Geometry check sheet. Reference: drawing and pictorial views, mm from the part's lowest x, y, z. A direction names the side the tool comes from. Give positions to 0.01 mm unless a question says otherwise; leave off trailing zeros. Order: outer loops, then holes, each group sorted by start corner. A loop starts at its lowest first (then second) coordinate and runs counter-clockwise, first axis right, second up.
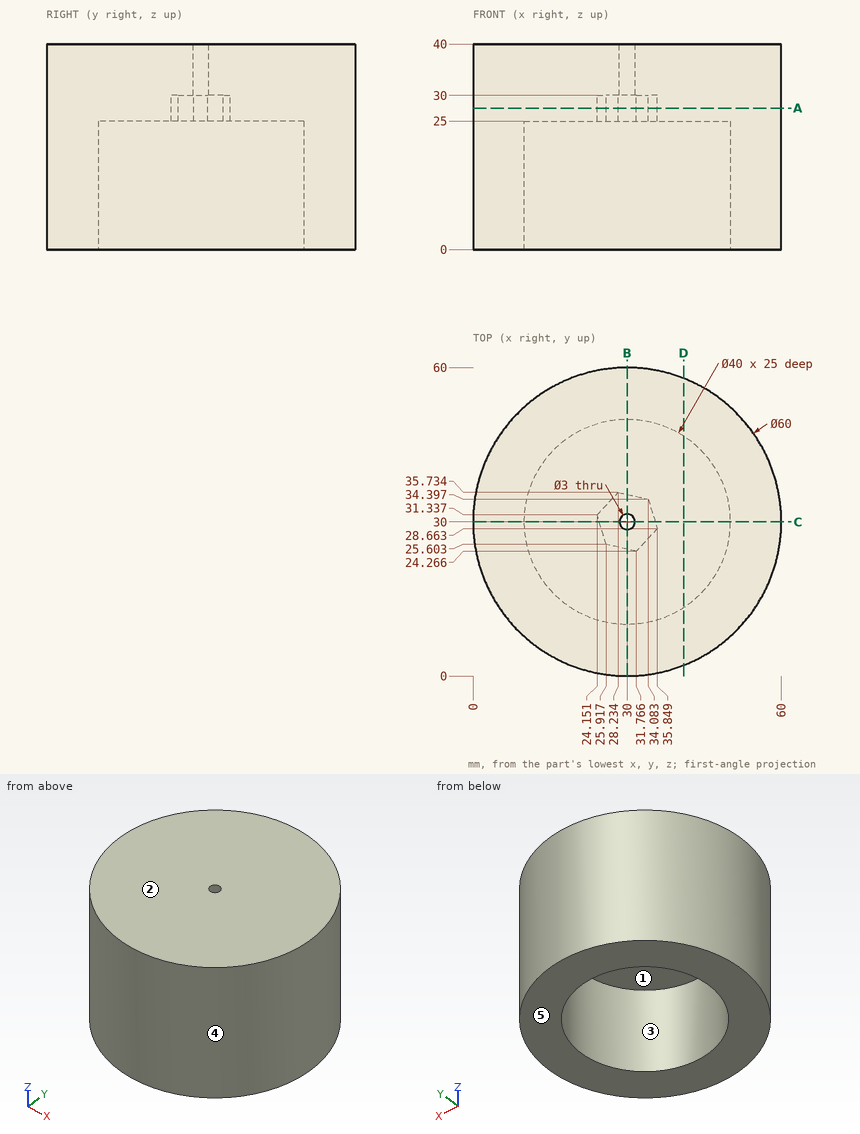
(1) Sectioned sample at B-B (x = 30). Enter the section's corners in (y, z).
(2) Sectioned sample at C-C (y = 30). Enter the section's corners in (x, z), plus the area to 3 significant figures.
(3) Thickness scan on L1, parallel to Y at x = 30, z = 8; L2, parallel to Z at x = 20.5, y = 32; L3, parallel to X at y = 21, z = 6.5. Record the ranges inside material, lowest first.
(4) Go/stop test with flat-tipped pins: P1, Ø5.5, axis at x = 29.5, y = 28.5, coming from the -Z side; P2, Ø5, axis at x = 31.5, z = 33.5, coming from the +Y side; P3, Ø6, axis at x = 21.5, z = 11, coming from the +Y side; P4, Ø2.5, axis at x = 30, y = 30, coming from the +Z side. Record where each tip stops, or that it passes through.
(5) Tool access check on the marked faces 1 and 2. Record the directions out of +Z, -Z, +X, -X, +Y, -Y that give a thin tool (end or side, any length) a straight path to the whole face; none if there is none.
(6) Sectioned sample at A-A (z = 27.5). Enter the section's corners in (x, y) (1 decimal), plus the area to 3 significant figures.
(7) Sectioned sample at D-D (x = 41). Enter the section's corners in (y, z).
(8) Release check for a two-part mould opening along Y. For the marked faces 3, 4 and 5 record: released by +Y, released by -Y, zero draft, split by the parting line, or undercut.
Values follow:
1. outline: (0, 0) - (10, 0) - (10, 25) - (24.67, 25) - (24.67, 30) - (28.5, 30) - (28.5, 40) - (0, 40) - close; (31.5, 30) - (35.33, 30) - (35.33, 25) - (50, 25) - (50, 0) - (60, 0) - (60, 40) - (31.5, 40) - close
2. outline: (0, 0) - (10, 0) - (10, 25) - (24.56, 25) - (24.56, 30) - (28.5, 30) - (28.5, 40) - (0, 40) - close; (31.5, 30) - (35.44, 30) - (35.44, 25) - (50, 25) - (50, 0) - (60, 0) - (60, 40) - (31.5, 40) - close
2. area: 1,320 mm2
3. L1: y = 0 to 10, 50 to 60
3. L2: z = 25 to 40
3. L3: x = 1.38 to 12.14, 47.86 to 58.62
4. P1: stops at z = 30
4. P2: stops at y = 60
4. P3: stops at y = 59.49
4. P4: passes through
5. face 1: -Z
5. face 2: +Z, +X, -X, +Y, -Y
6. outline: circle Ø60 at (30, 30); hole (24.2, 31.3) - (25.9, 25.6) - (31.8, 24.3) - (35.8, 28.7) - (34.1, 34.4) - (28.2, 35.7) - close
6. area: 2,730 mm2
7. outline: (2.09, 0) - (13.3, 0) - (13.3, 25) - (46.7, 25) - (46.7, 0) - (57.91, 0) - (57.91, 40) - (2.09, 40) - close
8. face 3: undercut
8. face 4: split by the parting line
8. face 5: zero draft
